Can you work these out from the drawing? Everything is in mm from the part's minimum corner. A direction names the side the tool comes from. Round coordinates to 2 decimals unless told otherwise and drop trailing zeros. Loops run counter-clockwise (first coordinate to the right, second up) from the corner with the lowest first, then second, coordinate; pieces in that order, holes last. Notation, with made-up numbers: (-7.5, 89) - (16.5, 89) arc R11 cw to (16.5, 98) - close; hole circle Ø6 at (39.25, 73.25). An arc over 180 degrees is marked (long way). Return JSON: item names as keys, results as strings. Group by question number.
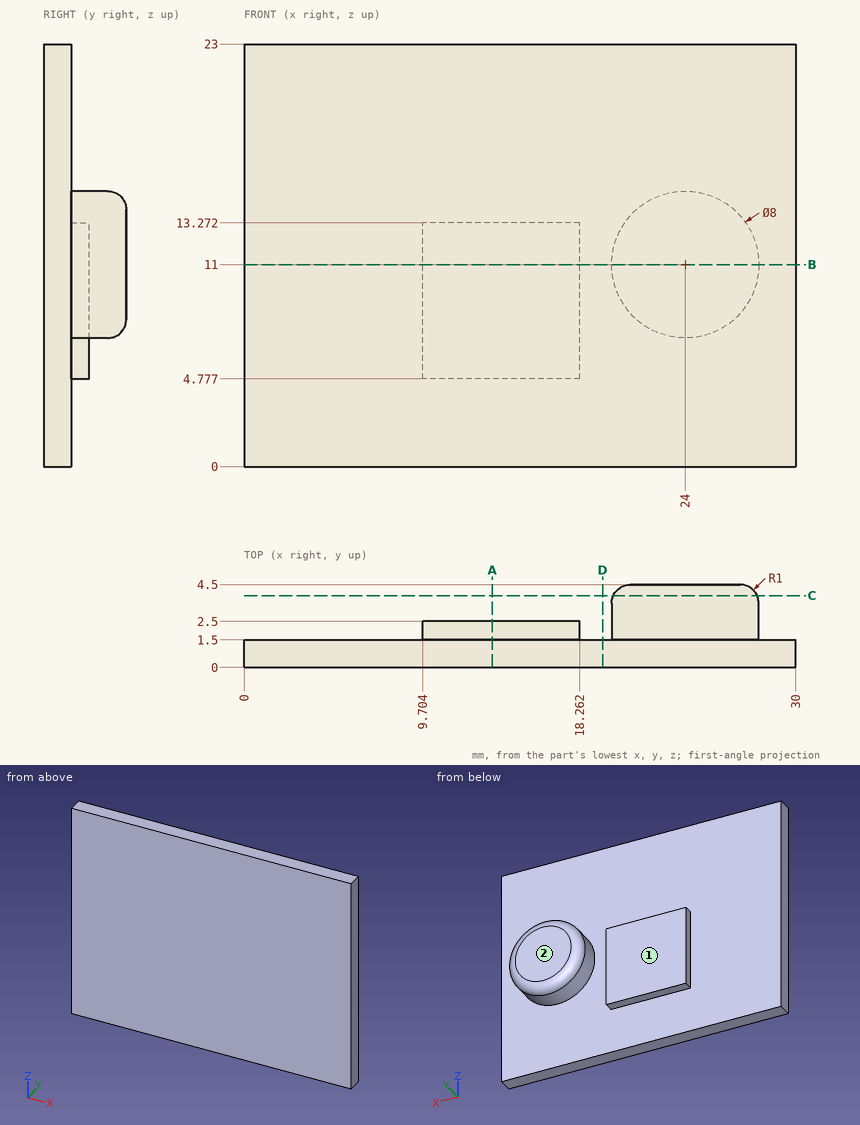
Q1. Imagine slicing it at D-D, the plane x = 19.5. List the corners of the cut face in (y, z) for me.
Q2. Will these pins go through, and if not, where does the flat tip stop? pin 1 Ø0.5 at (x, y) = (12.5, 2) entering from -Z; pin 2 Ø1.5 at (y, z) = (3, 9) entering from -X; pin 3 Ø2 at (x, z) = (8, 16) entering from +Y.
Q3. For the marked faces 1 and 2, which set-ups out of +Z, -Z, +X, -X, +Y, -Y let a thin tool reach every point of the face, with its end or its side?
Q4. Imagine slicing it at B-B, the plane z = 11. List the corners of the cut face in (x, y) for me (1 decimal).
Q5. Imagine slicing it at C-C, the plane y = 3.9. List the corners of the cut face in (x, z) for me, and give its area (3 significant figures).
Q6. Imagine slicing it at A-A, the plane x = 13.5. List the corners of the cut face in (y, z) for me.
Q7. Please list where these lines run through material, in increasing order: line 1 (Y direction, x = 13, z = 7.25); line 2 (Y direction, x = 23, z = 2.75); line 3 (X direction, y = 2.25, z = 8.5) (1 decimal).
Output values:
{
 "1": {"outline": "(0, 0) - (1.5, 0) - (1.5, 23) - (0, 23) - close"},
 "2": {"pin 1": "stops at z = 4.78", "pin 2": "stops at x = 9.7", "pin 3": "stops at y = 1.5"},
 "3": {"face 1": "+Z, -Z, -X, +Y", "face 2": "+Z, -Z, +X, -X, +Y"},
 "4": {"outline": "(0, 0) - (30, 0) - (30, 1.5) - (28, 1.5) - (28, 3.5) arc R1 ccw to (27, 4.5) - (21, 4.5) arc R1 ccw to (20, 3.5) - (20, 1.5) - (18.3, 1.5) - (18.3, 2.5) - (9.7, 2.5) - (9.7, 1.5) - (0, 1.5) - close"},
 "5": {"outline": "circle Ø7.83 at (24, 11)", "area": "48.2 mm^2"},
 "6": {"outline": "(0, 0) - (1.5, 0) - (1.5, 4.78) - (2.5, 4.78) - (2.5, 13.27) - (1.5, 13.27) - (1.5, 23) - (0, 23) - close"},
 "7": {"line 1": "y = 0 to 2.5", "line 2": "y = 0 to 1.5", "line 3": "x = 9.7 to 18.3, 20.9 to 27.1"}
}
